```python
from build123d import *

# Parameters (mm, degrees)
BOSS_EXTRUDE1_DEPTH = 11.1
CUT_EXTRUDE1_REACH  = 14.123
CUT_EXTRUDE2_DEPTH  = 4.75


with BuildPart() as part:
    # Sketch1 → Boss-Extrude1 (new body)
    with BuildSketch(Plane.XY):
        with BuildLine():
            Line((0, 0), (-3.095, 0))
            ThreePointArc((-3.095, 0), (-3.519264069, 0.175735931), (-3.695, 0.6))
            Line((-3.695, 0.6), (-3.695, 1.76))
            ThreePointArc((-3.695, 1.76), (-2.275, 3.18), (-0.855, 1.76))
            Line((-0.855, 1.76), (-0.855, 0.95))
            Line((-0.855, 0.95), (-1.355, 0.95))
            Line((-1.355, 0.95), (-1.355, 1.76))
            ThreePointArc((-1.355, 1.76), (-2.275, 2.68), (-3.195, 1.76))
            Line((-3.195, 1.76), (-3.195, 0.6))
            ThreePointArc((-3.195, 0.6), (-3.165710678, 0.529289322), (-3.095, 0.5))
            Line((-3.095, 0.5), (0, 0.5))
            Line((0, 0.5), (3.095, 0.5))
            ThreePointArc((3.095, 0.5), (3.165710678, 0.529289322), (3.195, 0.6))
            Line((3.195, 0.6), (3.195, 1.76))
            ThreePointArc((3.195, 1.76), (2.275, 2.68), (1.355, 1.76))
            Line((1.355, 1.76), (1.355, 0.95))
            Line((1.355, 0.95), (0.855, 0.95))
            Line((0.855, 0.95), (0.855, 1.76))
            ThreePointArc((0.855, 1.76), (2.275, 3.18), (3.695, 1.76))
            Line((3.695, 1.76), (3.695, 0.6))
            ThreePointArc((3.695, 0.6), (3.519264069, 0.175735931), (3.095, 0))
            Line((3.095, 0), (0, 0))
        make_face()
    extrude(amount=-BOSS_EXTRUDE1_DEPTH)

    # Sketch2 → Cut-Extrude1 (cut, up to next)
    with BuildSketch(Plane.XZ, mode=Mode.PRIVATE) as cut_extrude1_sk1:
        with BuildLine():
            Line((-3.095, 0), (-1.395, -1.7))
            Line((-1.395, -1.7), (-1.395, -3.238))
            ThreePointArc((-1.395, -3.238), (-1.933815367, -4.538815367), (-0.633, -4))
            Line((-0.633, -4), (0.633, -4))
            ThreePointArc((0.633, -4), (1.933815367, -4.538815367), (1.395, -3.238))
            Line((1.395, -3.238), (1.395, -1.7))
            Line((1.395, -1.7), (3.095, 0))
            Line((3.095, 0), (3.095, 0.537500588))
            Line((3.095, 0.537500588), (-3.095, 0.537500588))
            Line((-3.095, 0.537500588), (-3.095, 0))
        make_face()
    cut_extrude1_tool1 = extrude(cut_extrude1_sk1.sketch, amount=-CUT_EXTRUDE1_REACH, mode=Mode.PRIVATE) & part.part
    add(cut_extrude1_tool1.solids().sort_by_distance((0, 0, -1.705502))[0], mode=Mode.SUBTRACT)

    # Sketch3 → Cut-Extrude2 (cut)
    with BuildSketch(Plane.XY):
        Polygon((-3.695, 3.311724778), (3.695, 3.311724778), (3.695, 1.27), (3.095, 1.27), (3.095, 0.77), (-3.095, 0.77), (-3.095, 1.27), (-3.695, 1.27), align=None)
    extrude(amount=-CUT_EXTRUDE2_DEPTH, mode=Mode.SUBTRACT)


solid = part.part
```
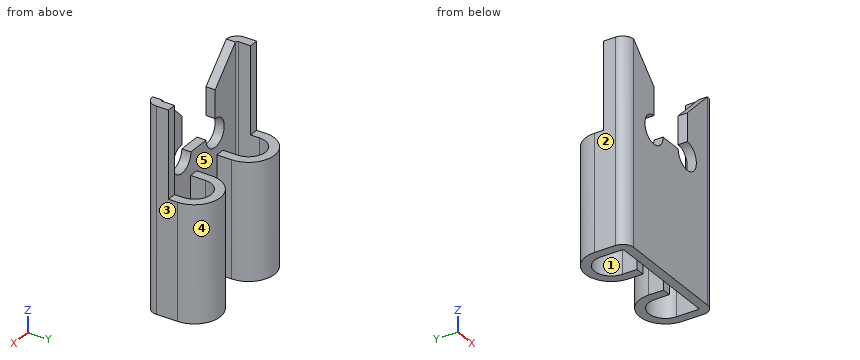
Geometry check sheet. Reference: the model listing, model coordinates, mm. Face numbers are marked on the shaded views. A direction names the side the tool comes from. Give positions to 0.01 mm unless a question says otherwise; leave off trailing zeros. Write each loop counter-clockwise with the first axis right and the second up, starting at its lowest first coordinate (ties: lowest second). Pieces come first, ordered by that corner, then holes.
1) Section check B-B, the plane x = 2.5. Record the boundary of the cut face in (y, z) (3 decimals).
2) Gauge pin test, flat ends, axial feed: pin 1 (0.6 mm diameter, centred on y = 0, z = -2, fed in from +X); pin 2 (1 mm diameter, centred on x = -2, z = -3.5, fed in from +Y). Record the tip position at first contact, or that the pin passes through.
3) Material ranges on L1, parallel to X at y = 1.3, z = -10.5 (3 decimals); L2, parallel to X at y = 2.25, z = -5.5; L3, parallel to Y at x = -2.25, z = -8.25, recorded low to high.
4) Access from +Z, -Z, +X, -X, +Y, -Y to the whole of each face (thin tool, end or side, straight path). Record for the marked faces 4 and 5.
5) Section check A-A, the plane y = 1.4. Record the boundary of the cut face in (x, z) (3 decimals).
6) Section check C-C, the plane z = -4.25. Record the boundary of the cut face in (x, y) (3 decimals), and give its area (3 significant figures).
7) Release check for a two-part mould opening along X. For the marked faces 1, 2 and 3 record: pulls with the +X half, pulls with the -X half, needs draft (parallel to the pull), parting line crosses it, or undercut.
8) Section check D-D, the plane y = 2.9. Record the boundary of the cut face in (x, z), and give its area (3 significant figures).
Computed:
1. outline: (0, -11.1) - (0.5, -11.1) - (0.5, -0.595) - (0, -0.595) - close; (2.652, -11.1) - (3.162, -11.1) - (3.162, -4.75) - (2.652, -4.75) - close
2. pin 1: stops at x = 3.61
2. pin 2: stops at y = 0.5
3. L1: x = -3.695 to -3.195, -1.355 to -0.855, 0.855 to 1.355, 3.195 to 3.695
3. L2: x = -3.61 to -3.05, -1.5 to -0.94, 0.94 to 1.5, 3.05 to 3.61
3. L3: y = 0 to 0.5, 2.68 to 3.18
4. face 4: +Z, -Z, +Y
4. face 5: +Z, -Z
5. outline: (-3.695, -11.1) - (-3.195, -11.1) - (-3.195, -4.75) - (-3.695, -4.75) - close; (-1.355, -11.1) - (-0.855, -11.1) - (-0.855, -4.75) - (-1.355, -4.75) - close; (0.855, -11.1) - (1.355, -11.1) - (1.355, -4.75) - (0.855, -4.75) - close; (3.195, -11.1) - (3.695, -11.1) - (3.695, -4.75) - (3.195, -4.75) - close
6. outline: (-3.695, 0.6) arc R0.6 ccw to (-3.095, 0) - (-2.115, 0) - (-2.115, 0.5) - (-3.095, 0.5) arc R0.1 cw to (-3.195, 0.6) - (-3.195, 1.27) - (-3.695, 1.27) - close; (-0.675, 0) - (0.675, 0) - (0.675, 0.5) - (-0.675, 0.5) - close; (2.115, 0) - (3.095, 0) arc R0.6 ccw to (3.695, 0.6) - (3.695, 1.27) - (3.195, 1.27) - (3.195, 0.6) arc R0.1 cw to (3.095, 0.5) - (2.115, 0.5) - close
6. area: 2.88 mm2
7. face 1: undercut
7. face 2: pulls with the -X half
7. face 3: pulls with the +X half
8. outline: (-3.12, -11.1) - (-1.43, -11.1) - (-1.43, -4.75) - (-3.12, -4.75) - close; (1.43, -11.1) - (3.12, -11.1) - (3.12, -4.75) - (1.43, -4.75) - close
8. area: 21.5 mm2
